The model under review builds one solid part; all positions refer to its coordinate system, in mm. A direction names the side the tool comes from. Round coordinates to 2 decimals unless told otherwise and drop trailing zeros. Order: outer loops, then holes, each group sorted by start corner. A loop starts at its lowest first (then second) coordinate and runs counter-clockwise, first axis right, second up.
1) Clearance check with flat-ended pins moving along their axes: P1, Ø2.5, axis at x = -78.5, z = 10.5, coming from the -Y side; P2, Ø1, axis at x = -105.5, z = 14, coming from the +Y side; P3, Ø1.5, axis at x = -84, y = 10.5, coming from the -Z side; P4, Ø10, axis at y = 41, z = 11.5, coming from the -X side. State where each tip first meets the part, or that it passes through.
2) To check wall thickness, follow L1, parallel to X at y = 49.5, z = 2.5; L2, parallel to Y at x = -213, z = 26.75. State the ranges of each line that lie inside material, in increasing order.
3) Consider section B-B (z = 25.25). Give the boundary of the cut face in (x, y).
4) Consider section C-C (x = -201). Give the boundary of the cut face in (y, z), then the cut area to 3 significant figures.
5) Machinability: for faces 5 (the face through (-84, 30, 15)), 6 (the face through (-145.75, 7.11, 14.79)), 7 (the face through (-75, -37, 15)), 8 (the face through (1, 60, 15)), which of the approach directions +Z, -Z, +X, -X, +Y, -Y give a long, thin tool a straight path to every point of the face, cutting with its end or side? Answer none if there is none.
6) Consider section A-A (y = -42.5). Give the boundary of the cut face in (x, z).
7) Mouldability with a two-part tool opening along Y and no side actions: class faces 1 (the face through (-155.68, -35.105, 14.79)), 2 (the face through (-192.17, 1.69, 14.79)), 3 (the face through (-49, 1, 0)), 4 (the face through (-116.973, 15.59, 14.79)) as pulls with the +Y half, pulls with the -Y half, needs draft (parallel to the pull), parting line crosses it, or undercut.
8) Consider section D-D (y = 38.5). Give the boundary of the cut face in (x, z), then the cut area to 3 significant figures.
from build123d import *

# Parameters (mm, degrees)
F1_DEPTH = 30


with BuildPart() as f1:
    # F0 (on Top) → F1 (new body)
    with BuildSketch(Plane.XY):
        Polygon((75, -60), (75, 60), (-75, 60), (-75, 30), (26.413014, 30), (26.413014, -15), (-75, -15), (-75, -60), align=None)
        Polygon((26.413014, 30), (-75, 30), (-93.586986, 30), (-119.013755, 22.697953), (-114.873411, 8.280687), (-143.707943, 0), (-147.848286, 14.417266), (-237.759645, -11.403435), (-225.338615, -54.655232), (-84.043801, -15), (-75, -15), (26.413014, -15), align=None)
    extrude(amount=F1_DEPTH)


solid = f1.part
Answer below:
1. P1: stops at y = -15
1. P2: stops at y = 26.72
1. P3: stops at z = 0
1. P4: stops at x = -75
2. L1: x = -75 to 75
2. L2: y = -51.19 to -4.29
3. outline: (-237.76, -11.4) - (-225.34, -54.66) - (-84.04, -15) - (-75, -15) - (-75, -60) - (75, -60) - (75, 60) - (-75, 60) - (-75, 30) - (-93.59, 30) - (-119.01, 22.7) - (-114.87, 8.28) - (-143.71, 0) - (-147.85, 14.42) - close
4. outline: (-47.82, 0) - (-0.85, 0) - (-0.85, 30) - (-47.82, 30) - close
4. area: 1,410 mm2
5. face 5: +Z, -Z, -X, +Y
5. face 6: +Z, -Z, +Y
5. face 7: +Z, -Z, -Y
5. face 8: +Z, -Z, +X, -X, +Y
6. outline: (-228.83, 0) - (-182.03, 0) - (-182.03, 30) - (-228.83, 30) - close; (-75, 0) - (75, 0) - (75, 30) - (-75, 30) - close
7. face 1: pulls with the -Y half
7. face 2: pulls with the +Y half
7. face 3: needs draft
7. face 4: undercut
8. outline: (-75, 0) - (75, 0) - (75, 30) - (-75, 30) - close
8. area: 4,500 mm2
